Can you work these out from the model? Positions are in its coordinate system, mm. A direction names the side the tool comes from. Give positions to 0.01 mm unless a question says otherwise; leave off trailing zeros. Order: outer loops, then holes, each group sorted by start corner. A loop starts at its lowest first (then second) coordinate and runs counter-clockwise, first axis right, second up. Notation, with made-up numbers: (7.5, 71.5) -> (25.5, 71.5) arc R23 cw to (25.5, 90.5) -> close; hole circle Ø6 at (-14.75, -24.75). An arc over 180 degrees is marked (long way). Answer as CSV lines item,"result".
```python
from build123d import *

# Parameters (mm, degrees)
CROQUIS2_R            = 11.708753873
CROQUIS2_R_2          = 11.163314546
CORTAR_EXTRUIR1_DEPTH = 40
CHAFL_N1_SIZE         = 5


with BuildPart() as part:
    # Croquis1 → Revolución1 (revolve)
    with BuildSketch(Plane(origin=(0, 0, 0), x_dir=(0, 0, -1), z_dir=(1, 0, 0))):
        with BuildLine():
            Line((0, 0), (100, 0))
            Line((100, 0), (100, 22.244599069))
            Line((100, 22.244599069), (65.358062391, 22.244599069))
            ThreePointArc((65.358062391, 22.244599069), (40.58262282, 28.815543652), (22.320043888, 46.801035845))
            Line((22.320043888, 46.801035845), (22.320043888, 80))
            Line((22.320043888, 80), (14.629845341, 80))
            Line((14.629845341, 80), (14.629845341, 92.520583479))
            ThreePointArc((14.629845341, 92.520583479), (35.962664377, 133.682908793), (0, 162.942316925))
            Line((0, 162.942316925), (0, 0))
        make_face()
    revolve(axis=Axis((0, 0, 0), (0, 1, 0)))

    # Croquis2 → Cortar-Extruir1 (cut)
    with BuildSketch(Plane(origin=(0, 22.244599069, 0), x_dir=(1, 0, 0), z_dir=(0, 1, 0))):
        with Locations((0, -81.89901044)):
            Circle(CROQUIS2_R)
        with Locations((0, 81.054690745)):
            Circle(CROQUIS2_R_2)
    extrude(amount=-CORTAR_EXTRUIR1_DEPTH, mode=Mode.SUBTRACT)

    # Chaflán1
    chafl_n1_edges = [part.edges().sort_by_distance(p)[0] for p in [
        (0, 22.244599069, 100),
    ]]
    chamfer(chafl_n1_edges, length=CHAFL_N1_SIZE)


solid = part.part
```
Item 1: Imagine slicing it at D-D, the plane y = 131. Please give me the cut outline in (x, z).
Numbers:
outline,"circle Ø72.83 at (0, 0)"
Item 2: Imagine slicing it at C-C, the plane y = 85. Please give me the cut outline in (x, z).
Numbers:
outline,"circle Ø29.26 at (0, 0)"
Item 3: Imagine slicing it at A-A, the plane x = 0. Please give me the cut outline in (y, z), then the cut area to 3 significant figures.
Numbers:
outline,"(0, -100) -> (17.24, -100) -> (22.24, -95) -> (22.24, -92.22) -> (0, -92.22) -> close; (0, -69.89) -> (22.24, -69.89) -> (22.24, -65.36) arc R49.99 cw to (46.8, -22.32) -> (80, -22.32) -> (80, -14.63) -> (92.52, -14.63) arc R36.73 ccw (long way) to (92.52, 14.63) -> (80, 14.63) -> (80, 22.32) -> (46.8, 22.32) arc R49.99 cw to (22.24, 65.36) -> (22.24, 70.19) -> (0, 70.19) -> close; (0, 93.61) -> (22.24, 93.61) -> (22.24, 95) -> (17.24, 100) -> (0, 100) -> close"
area,"11,100 mm²"
Item 4: Please list where these lines run through material, in increasing order: line 1 along Z through (x, y) = (0, 15); line 2 along Y through (x, z) = (-46.5, -71); line 3 along Z through (x, y) = (-8, 7).
Numbers:
line 1,"z = -100 to -92.22, -69.89 to 70.19, 93.61 to 100"
line 2,"y = 0 to 22.24"
line 3,"z = -99.68 to -88.84, -73.27 to 73.35, 90.45 to 99.68"
Item 5: For faces 5 (the conical face through (-4.19, 22, 95.15)), 6 (the cylindrical face through (14.282, 86.348, 3.171)), which set-ups out of +Z, -Z, +X, -X, +Y, -Y let a thin tool reach every point of the face, with its end or its side?
Numbers:
face 5,"+Y"
face 6,"none"
Item 6: Imagine slicing it at B-B, the plane z = 0. Please give me the cut outline in (x, y).
Numbers:
outline,"(-100, 0) -> (100, 0) -> (100, 17.24) -> (95, 22.24) -> (65.36, 22.24) arc R49.99 cw to (22.32, 46.8) -> (22.32, 80) -> (14.63, 80) -> (14.63, 92.52) arc R36.73 ccw (long way) to (-14.63, 92.52) -> (-14.63, 80) -> (-22.32, 80) -> (-22.32, 46.8) arc R49.99 cw to (-65.36, 22.24) -> (-95, 22.24) -> (-100, 17.24) -> close"
Item 7: We'd pull the mould along Z, two halves only. Please class faces 1 (the cylindrical face through (-2.54, 11.28, 93.33)), 2 (the flat face through (-22, 22.245, -62)), 3 (the cylindrical face through (-30.04, 8.74, -95.38)), 4 (the cylindrical face through (-2.42, 11.278, -70.157)): released by +Z, released by -Z, zero draft, split by the parting line, or undercut.
Numbers:
face 1,"undercut"
face 2,"zero draft"
face 3,"split by the parting line"
face 4,"undercut"
Item 8: For pin 1 (6 mm diameter, centred on y = 74, z = -18, fed in from +X); pin 2 (2 mm diameter, centred on x = -41, z = 21.5, fed in from -Y); pin 3 (12 mm diameter, centred on y = 96, z = 11.5, fed in from -X); pin 4 (12 mm diameter, centred on x = 74, z = 52.5, fed in from +Y), each with a flat end and sliding along its axis, tell me the tip position at first contact or that it passes through.
Numbers:
pin 1,"stops at x = 16.53"
pin 2,"stops at y = 0"
pin 3,"stops at x = -25.61"
pin 4,"stops at y = 22.24"
